from build123d import *

# Parameters (mm, degrees)
F0_W       = 19.05
F0_H       = 19.05
F1_DEPTH   = 6.35
F3_DEPTH   = 12.7
F7_D       = 2.9
F7_ON_F6_D = 2.9
F7_ON_F5_D = 2.9
F8_R       = 1.5875
F9_SIZE    = 0.508


with BuildPart() as f1:
    # F0 (on Top) → F1 (new body)
    with BuildSketch(Plane.XY):
        with Locations((9.525, 9.525)):
            Rectangle(F0_W, F0_H)
    extrude(amount=F1_DEPTH)

    # F2 (on face) → F3 (join)
    with BuildSketch(Plane.XY.offset(6.35)):
        Polygon((6.35, 19.05), (0, 19.05), (0, 0), (19.05, 0), (19.05, 6.35), (6.35, 6.35), align=None)
    extrude(amount=F3_DEPTH)

    # F7 (through all)
    with Locations(Plane.YZ.offset(6.35)):
        with Locations((12.7, 12.7)):
            Hole(F7_D / 2)

    # F7 on F6 (through all)
    with Locations(Plane(origin=(0, 6.35, 0), x_dir=(-1, 0, 0), z_dir=(0, 1, 0))):
        with Locations((-12.7, 12.7)):
            Hole(F7_ON_F6_D / 2)

    # F7 on F5 (through all)
    with Locations(Plane.XY.offset(6.35)):
        with Locations((12.7, 12.7)):
            Hole(F7_ON_F5_D / 2)

    # F8
    f8_edges = [f1.edges().sort_by_distance(p)[0] for p in [
        (6.35, 6.35, 12.7),
    ]]
    fillet(f8_edges, radius=F8_R)

    # F9
    f9_edges = [f1.edges().sort_by_distance(p)[0] for p in [
        (19.05, 19.05, 3.175),
        (12.7, 19.05, 6.35),
        (6.35, 19.05, 12.7),
        (0, 19.05, 9.525),
        (3.175, 19.05, 19.05),
        (6.35, 13.49375, 19.05),
        (19.05, 6.35, 12.7),
        (19.05, 12.7, 6.35),
        (19.05, 0, 9.525),
        (19.05, 3.175, 19.05),
        (13.49375, 6.35, 19.05),
        (6.814968, 6.814968, 19.05),
        (9.525, 0, 19.05),
        (0, 9.525, 19.05),
        (0, 0, 9.525),
        (19.05, 9.525, 0),
        (9.525, 19.05, 0),
        (0, 9.525, 0),
        (9.525, 0, 0),
    ]]
    chamfer(f9_edges, length=F9_SIZE)


solid = f1.part
Geometry check sheet. Reference: the model listing, model coordinates, mm. A direction names the side the tool comes from. Give positions to 0.01 mm unless a question says otherwise; leave off trailing zeros. Loops run counter-clockwise (first coordinate to the right, second up) from the corner with the lowest first, then second, coordinate; pieces in that order, holes last. Notation, with made-up numbers: (67, 31) -> (88, 31) arc R16 ccw to (88, 50) -> close; hole circle Ø11 at (54, 27). An arc over 180 degrees is marked (long way). Answer in a Markdown table with one row per item. Add a question column.
1) Material ranges on probe 1 along Z at (x, y) = (17.5, 14.75); probe 2 along Z at (x, y) = (13, 1.25), recorded low to high. Write a range as from..to.
2) Cross-section at C-C on z = 12.7. State how many separate pieces and enclosed holes the cut face has, and give its area (3 significant figures).
3) Draft check along Y on faces 1 (the face through (14.5, 6.35, 12.4)), 2 (the face through (0, 10, 9)), 3 (the face through (11.92, 13.92, 3.13)), 4 (the face through (3.13, 11.92, 13.92)). Enter one of: pulls with the +Y half, pulls with the -Y half, needs draft (parallel to the pull), parting line crosses it, or undercut.
4) Gauge pin test, flat ends, axial feed: P1, Ø3, axis at x = 10, z = 11, coming from the +Y side; P2, Ø5.5, axis at y = 14.5, z = 13, coming from the +X side. Record the tip position at first contact, or that the pin passes through.
5) Cross-section at A-A on y = 12.7. Record the boundary of the cut face in (x, z).
6) Set-up check for faces 5 (the face through (6.35, 14.3, 12.4)), 6 (the face through (9, 0, 9)): record each of +Z, -Z, +X, -X, +Y, -Y from which the full face is reachable in a straight line by a thin tool's end or side.
Outcome:
| question | item | result |
|---|---|---|
| 1 | probe 1 | z = 0..6.35 |
| 1 | probe 2 | z = 0..11.28, 14.12..19.05 |
| 2 | separate pieces | 3 |
| 2 | enclosed holes | 0 |
| 2 | area | 165 mm^2 |
| 3 | face 1 | pulls with the +Y half |
| 3 | face 2 | needs draft |
| 3 | face 3 | undercut |
| 3 | face 4 | undercut |
| 4 | P1 | stops at y = 6.35 |
| 4 | P2 | stops at x = 6.35 |
| 5 | outline | (0, 0.51) -> (0.51, 0) -> (11.25, 0) -> (11.25, 6.35) -> (6.35, 6.35) -> (6.35, 11.25) -> (0, 11.25) -> close; (0, 14.15) -> (6.35, 14.15) -> (6.35, 18.54) -> (5.84, 19.05) -> (0.51, 19.05) -> (0, 18.54) -> close; (14.15, 0) -> (18.54, 0) -> (19.05, 0.51) -> (19.05, 5.84) -> (18.54, 6.35) -> (14.15, 6.35) -> close |
| 6 | face 5 | +Z, +X, +Y |
| 6 | face 6 | +Z, -Z, +X, -X, -Y |
